Build history of the part. All positions in model axes, mm. Face numbers are marked on the shaded views. A direction names the side the tool comes from. Round coordinates to 2 decimals unless told otherwise and drop trailing zeros. Order: outer loops, then holes, each group sorted by start corner. A loop starts at its lowest first (then second) coordinate and runs counter-clockwise, first axis right, second up. Notation, with made-up numbers: (64, 57.5) - (91, 57.5) arc R11 ccw to (91, 78.5) - close; hole circle Ø10 at (18.25, 45). An arc over 180 degrees is marked (long way). Write each question's results on one line, items separated by ' | '. Start each with the question number.
```python
from build123d import *

# Parameters (mm, degrees)
F0_R           = 37.5
F1_DEPTH       = 12.7
F3_D           = 18
F5_D           = 6.5
F5_CBORE_D     = 12.7
F5_CBORE_DEPTH = 10


# Not quite as in the source:
# - a length typed as a fraction of an inch, garbled in the dataset ("3 / 203.2 mm" for 3/8 in), is restored


with BuildPart() as f1:
    # F0 (on Top) → F1 (new body)
    with BuildSketch(Plane.XY):
        Circle(F0_R)
    extrude(amount=F1_DEPTH)

    # F3 (through all)
    with Locations(Plane.XY.offset(12.7)):
        with Locations((0, 0)):
            Hole(F3_D / 2)

    # F5 (through all)
    with Locations(Plane.XY.offset(12.7)):
        with Locations((0, 30), (25.9807621135, 15), (25.9807621135, -15), (0, -30), (-25.9807621135, -15), (-25.9807621135, 15)):
            CounterBoreHole(F5_D / 2, F5_CBORE_D / 2, F5_CBORE_DEPTH)


solid = f1.part
```
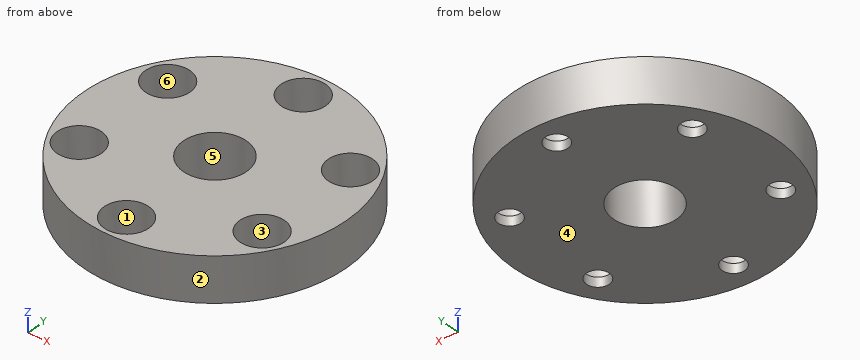
1. Cut at A-A (y = 30). List the corners of the cut face in (x, z).
2. Flat gauge pins, fed straight in: pin 1 Ø2 at (x, z) = (-4.5, 11) entering from +Y; pin 2 Ø2 at (y, z) = (27.5, 7) entering from +X; pin 3 Ø11.5 at (x, y) = (-25.98, -15) entering from +Z; pin 4 Ø2 at (x, y) = (-28, -27) entering from -Z. Where does each tip first touch, or does it go through?
3. Cut at C-C (y = -16.5). List the corners of the cut face in (x, z).
4. Cut at D-D (z = 10.75). List the corners of the cut face in (x, y).
5. Wall check: line 1 (Y direction, x = 0, z = 1.85); line 2 (Y direction, x = -28.5, z = 1.25); line 3 (X direction, y = -16, z = 7.5). Give the ranges that are in metal, low to high. Write a range as from..to.
6. 3-axis set-ups, long thin cutter, end or side, ignore diameter. For the marked faces 5 and 6: which of +Z, -Z, +X, -X, +Y, -Y reach the whole face in a straight line?
7. Mould opens along Y. For the marked faces 1, 2, 3 and 4 say: pulls with the +Y half, pulls with the -Y half, needs draft (parallel to the pull), parting line crosses it, or undercut.
8. Cut at B-B (x = 0). List the corners of the cut face in (y, z), plus the area to 3 significant figures.
A:
1) outline: (-22.5, 0) - (-3.25, 0) - (-3.25, 2.7) - (-6.35, 2.7) - (-6.35, 12.7) - (-22.5, 12.7) - close; (3.25, 0) - (22.5, 0) - (22.5, 12.7) - (6.35, 12.7) - (6.35, 2.7) - (3.25, 2.7) - close
2) pin 1: stops at y = 37.34 | pin 2: stops at x = 26.53 | pin 3: stops at z = 2.7 | pin 4: passes through
3) outline: (-33.67, 0) - (-28.86, 0) - (-28.86, 2.7) - (-32.15, 2.7) - (-32.15, 12.7) - (-33.67, 12.7) - close; (-23.1, 0) - (23.1, 0) - (23.1, 2.7) - (19.81, 2.7) - (19.81, 12.7) - (-19.81, 12.7) - (-19.81, 2.7) - (-23.1, 2.7) - close; (28.86, 0) - (33.67, 0) - (33.67, 12.7) - (32.15, 12.7) - (32.15, 2.7) - (28.86, 2.7) - close
4) outline: circle Ø75 at (0, 0); hole circle Ø12.7 at (-25.98, -15); hole circle Ø12.7 at (-25.98, 15); hole circle Ø18 at (0, 0); hole circle Ø12.7 at (0, -30); hole circle Ø12.7 at (0, 30); hole circle Ø12.7 at (25.98, -15); hole circle Ø12.7 at (25.98, 15)
5) line 1: y = -37.5..-33.25, -26.75..-9, 9..26.75, 33.25..37.5 | line 2: y = -24.37..-17.05, -12.95..12.95, 17.05..24.37 | line 3: x = -33.92..-32.25, -19.71..19.71, 32.25..33.92
6) face 5: +Z, -Z | face 6: +Z
7) face 1: undercut | face 2: parting line crosses it | face 3: undercut | face 4: needs draft
8) outline: (-37.5, 0) - (-33.25, 0) - (-33.25, 2.7) - (-36.35, 2.7) - (-36.35, 12.7) - (-37.5, 12.7) - close; (-26.75, 0) - (-9, 0) - (-9, 12.7) - (-23.65, 12.7) - (-23.65, 2.7) - (-26.75, 2.7) - close; (9, 0) - (26.75, 0) - (26.75, 2.7) - (23.65, 2.7) - (23.65, 12.7) - (9, 12.7) - close; (33.25, 0) - (37.5, 0) - (37.5, 12.7) - (36.35, 12.7) - (36.35, 2.7) - (33.25, 2.7) - close | area: 435 mm^2
